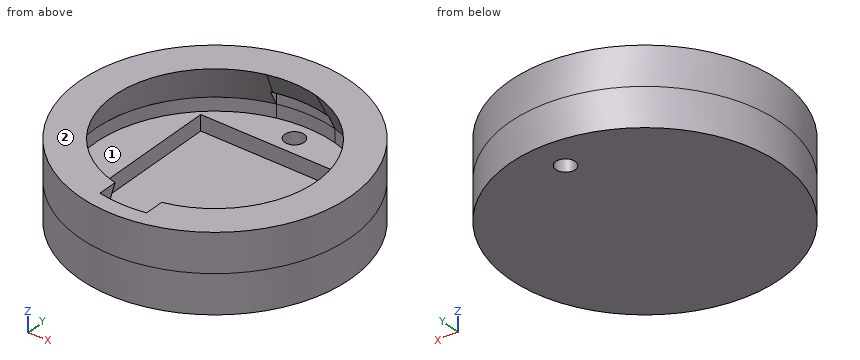
```python
from build123d import *

# Parameters (mm, degrees)
F0_R      = 35
F1_DEPTH  = 10
F2_R      = 2.5
F3_DEPTH  = 3.4
F4_DEPTH  = 10.001
F5_DEPTH  = 7.4
F2_R_2    = 35
F6_DEPTH  = 10
F6_TAPER  = -26
F7_R      = 39.8773258857
F7_R_2    = 35
F8_DEPTH  = 20.001
F9_DEPTH  = 4
F10_DEPTH = 10.0010001


# Not quite as in the source:
# - a feature names something its author has since deleted; it is built from what else it names


with BuildPart() as f1:
    # F0 (on Top) → F1 (new body)
    with BuildSketch(Plane.XY):
        Circle(F0_R)
    extrude(amount=F1_DEPTH)

    # F2 (on face) → F3 (cut)
    with BuildSketch(Plane.XY.offset(10)):
        with BuildLine():
            Line((7.5, 21.7), (7.5, 30.0790624854))
            ThreePointArc((7.5, 30.0790624854), (0, 31), (-7.5, 30.0790624854))
            Line((-7.5, 30.0790624854), (-7.5, 21.7))
            Line((-7.5, 21.7), (7.5, 21.7))
        make_face()
        with Locations((0, 26.35)):
            Circle(F2_R, mode=Mode.SUBTRACT)
        with BuildLine():
            Line((-7.5, 21.7), (-7.5, 30.0790624854))
            ThreePointArc((-7.5, 30.0790624854), (-30.9904741103, -0.7684493597), (-6, -30.4138126515))
            Line((-6, -30.4138126515), (-6, -21.7))
            Line((-6, -21.7), (-20.5, -21.7))
            Line((-20.5, -21.7), (-20.5, 21.7))
            Line((-20.5, 21.7), (-7.5, 21.7))
        make_face()
        with BuildLine():
            ThreePointArc((-6, -30.4138126515), (0, -31), (6, -30.4138126515))
            Line((6, -30.4138126515), (6, -21.7))
            Line((6, -21.7), (-6, -21.7))
            Line((-6, -21.7), (-6, -30.4138126515))
        make_face()
        with BuildLine():
            ThreePointArc((6, -30.4138126515), (23.9478600297, -19.685019685), (31, 0))
            ThreePointArc((31, 0), (24.4284670006, 19.085334684), (7.5, 30.0790624854))
            Line((7.5, 30.0790624854), (7.5, 21.7))
            Line((7.5, 21.7), (20.5, 21.7))
            Line((20.5, 21.7), (20.5, -21.7))
            Line((20.5, -21.7), (6, -21.7))
            Line((6, -21.7), (6, -30.4138126515))
        make_face()
    extrude(amount=-F3_DEPTH, mode=Mode.SUBTRACT)

    # F2 (on face) → F4 (cut, through all)
    with BuildSketch(Plane.XY.offset(10)):
        with Locations((0, 26.35)):
            Circle(F2_R)
    extrude(amount=-F4_DEPTH, mode=Mode.SUBTRACT)

    # F2 (on face) → F5 (cut)
    with BuildSketch(Plane.XY.offset(10)):
        Polygon((20.5, 21.7), (7.5, 21.7), (7.5, 20.0790624854), (0, 20.0790624854), (-7.5, 20.0790624854), (-7.5, 21.7), (-20.5, 21.7), (-20.5, -21.7), (-6, -21.7), (-6, -20.4138126515), (0, -20.4138126515), (6, -20.4138126515), (6, -21.7), (20.5, -21.7), align=None)
        Polygon((7.5, 20.0790624854), (7.5, 21.7), (-7.5, 21.7), (-7.5, 20.0790624854), (0, 20.0790624854), align=None)
        Polygon((-6, -21.7), (6, -21.7), (6, -20.4138126515), (0, -20.4138126515), (-6, -20.4138126515), align=None)
    extrude(amount=-F5_DEPTH, mode=Mode.SUBTRACT)

    # F2 (on face) → F6 (join)
    with BuildSketch(Plane.XY.offset(10)):
        Circle(F2_R_2)
        with BuildLine():
            ThreePointArc((7.5, 30.0790624854), (24.4284670006, 19.085334684), (31, 0))
            ThreePointArc((31, 0), (23.9478600297, -19.685019685), (6, -30.4138126515))
            ThreePointArc((6, -30.4138126515), (0, -31), (-6, -30.4138126515))
            ThreePointArc((-6, -30.4138126515), (-30.9904741103, -0.7684493597), (-7.5, 30.0790624854))
            ThreePointArc((-7.5, 30.0790624854), (0, 31), (7.5, 30.0790624854))
        make_face(mode=Mode.SUBTRACT)
    extrude(amount=F6_DEPTH, taper=F6_TAPER)

    # F7 (on face) → F8 (cut, through all)
    with BuildSketch(Plane.XY.offset(20)):
        Circle(F7_R)
        Circle(F7_R_2, mode=Mode.SUBTRACT)
    extrude(amount=-F8_DEPTH, mode=Mode.SUBTRACT)

    # F2 (on face) → F9 (cut)
    with BuildSketch(Plane.XY.offset(10)):
        with BuildLine():
            Line((7.5, 21.7), (7.5, 30.0790624854))
            ThreePointArc((7.5, 30.0790624854), (0, 31), (-7.5, 30.0790624854))
            Line((-7.5, 30.0790624854), (-7.5, 21.7))
            Line((-7.5, 21.7), (7.5, 21.7))
        make_face()
        with Locations((0, 26.35)):
            Circle(F2_R, mode=Mode.SUBTRACT)
        Polygon((7.5, 20.0790624854), (7.5, 21.7), (-7.5, 21.7), (-7.5, 20.0790624854), (0, 20.0790624854), align=None)
        with Locations((0, 26.35)):
            Circle(F2_R)
    extrude(amount=F9_DEPTH, mode=Mode.SUBTRACT)

    # F2 (on face) → F10 (cut, through all)
    with BuildSketch(Plane.XY.offset(10)):
        with BuildLine():
            ThreePointArc((-6, -30.4138126515), (0, -31), (6, -30.4138126515))
            Line((6, -30.4138126515), (6, -21.7))
            Line((6, -21.7), (-6, -21.7))
            Line((-6, -21.7), (-6, -30.4138126515))
        make_face()
        Polygon((-6, -21.7), (6, -21.7), (6, -20.4138126515), (0, -20.4138126515), (-6, -20.4138126515), align=None)
    extrude(amount=F10_DEPTH, mode=Mode.SUBTRACT)


solid = f1.part
```
Input: part model. Units: mm. Frame: model coordinates. Face numbers are marked on the shaded views. Round coordinates to 2 decimals unless told otherwise and drop trailing zeros. Write each loop counter-clockwise with the first axis right and the second up, starting at its lowest first coordinate (ties: lowest second). Pieces come first, ordered by that corner, then holes. Notation, with made-up numbers: M 44.25,72.5 L 57.25,72.5 A22 cw 57.25,106.5 Z; hole C -13,-37 d10. An arc over 180 degrees is marked long. Write each question's results on one line, items separated by ' | '.
Q1. Section query B-B (y = 0). Return loops of the section in (x, z), and give its area (3 significant figures).
Results:
outline: M -35,0 L 35,0 L 35,20 L 26.12,20 L 31,10 L 31,6.6 L 20.5,6.6 L 20.5,2.6 L -20.5,2.6 L -20.5,6.6 L -31,6.6 L -31,10 L -26.12,20 L -35,20 Z | area: 454 mm^2
Q2. Pin query (flat end, axial travel): P1, Ø0.6, axis at y = 28.5, z = 12, coming from the +X side; P2, Ø1.5, axis at x = -1, y = 30, coming from the -Z side; P3, Ø4.5, axis at y = -2.5, z = 4, coming from the +X side; P4, Ø4.5, axis at x = 0, y = 26.35, coming from the -Z side. Return the tip coordinate at first contact, or that it passes through.
Results:
P1: stops at x = 20.73 | P2: stops at z = 0 | P3: stops at x = 35 | P4: stops at z = 14.92
Q3. Draft query along Y for the marked faces 1 and 2. Return one class per face: released by +Y, released by -Y, zero draft, split by the parting line, or undercut.
Results:
face 1: undercut | face 2: zero draft
Q4. Line query: line 1 along Y through (x, z) = (0, 5); line 2 along Y through (x, z) = (0.5, 11.5); line 3 along Z through (x, y) = (4, -30). Output: solid intervals per line, ascending.
Results:
line 1: y = -35 to -21.7, 21.7 to 23.85, 28.85 to 35 | line 2: y = -35 to -31, 31 to 35 | line 3: z = 0 to 6.6
Q5. Section query C-C (z = 17.75). Return loops of the section in (x, y).
Results:
outline: C 0,0 d70; hole M -6,-30.41 A31 ccw 6,-30.41 L 6,-26.55 A27.22 ccw long -6,-26.55 Z
Q6. Section query A-A (x = 0). Return loops of the section in (y, z).
Results:
outline: M -35,0 L 23.85,0 L 23.85,6.6 L 21.7,6.6 L 21.7,2.6 L -21.7,2.6 L -21.7,6.6 L -31,6.6 L -31,20 L -35,20 Z; M 26.12,20 L 29.05,14 L 31,14 L 31,6.6 L 28.85,6.6 L 28.85,0 L 35,0 L 35,20 Z
